Could you check a few things on this drawing? It's one solid part, dimensions in mm from its lowest x, y, z. A direction names the side the tool comes from. Give positions to 0.01 mm unless a question says otherwise; leave off trailing zeros. Order: outer loops, then holes, each group sorted by start corner. A loop starts at its lowest first (then second) coordinate and runs counter-clockwise, first axis right, second up. Notation, with made-up numbers: M 74,-28.75 L 116,-28.75 A24 cw 116,7.25 Z; hole C 4,12 d9. An arc over 180 degrees is marked long. Return JSON: item names as keys, results as strings. Group by question number.
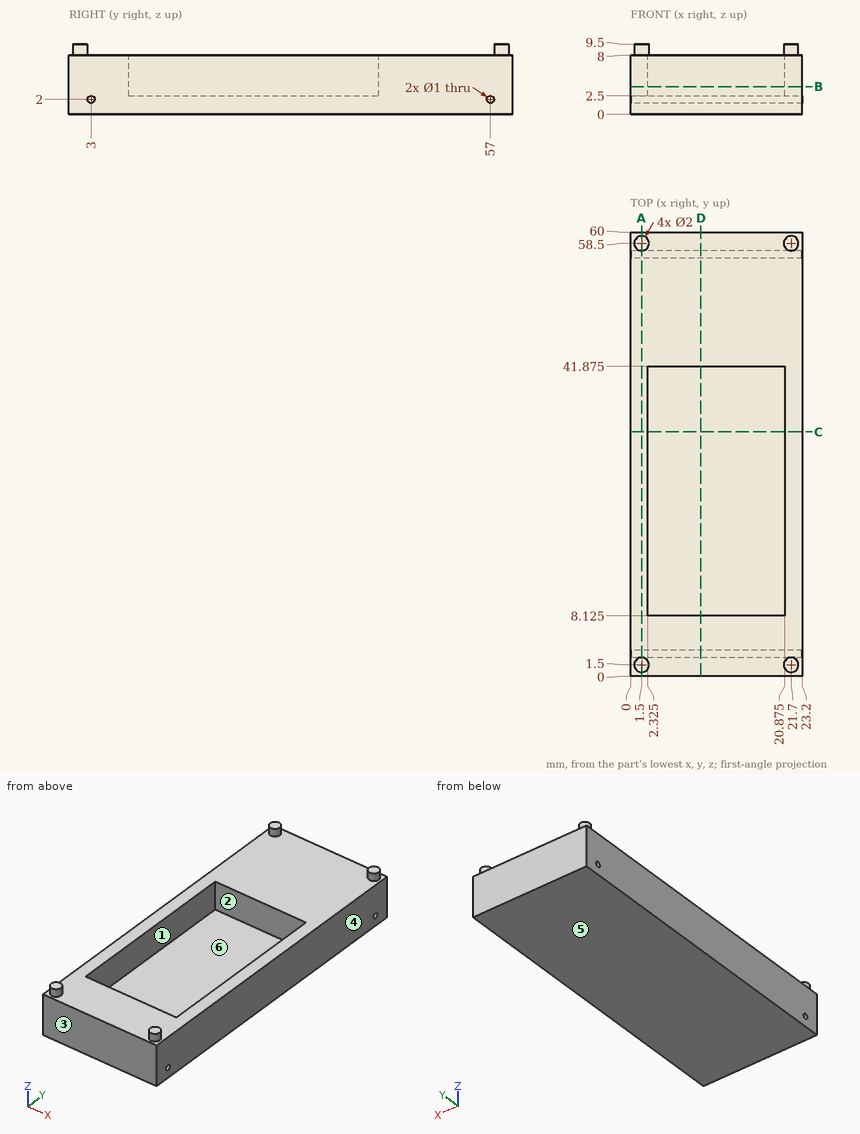
1. For pin 1 (4 mm diameter, centred on x = 16.5, y = 12.5, fed in from +Z), with a flat end and sliding along its axis, tell me the tip position at first contact or that it passes through.
2. I need wall thicknesses on L1, parallel to Y at x = 14.5, z = 2; L2, parallel to X at y = 18.5, z = 6 (3 decimals); L3, parallel to Y at x = 17.25, z = 7.5 (3 decimals). Which ranges of each line are inside material? Lowest first, please. Write a range as from..to.
3. If we mould it in two halves opening along Y, with no side actions, what happens to the marked faces 1, 2, 3 and 4? For each: pulls with the +Y half, pulls with the -Y half, needs draft (parallel to the pull), parting line crosses it, or undercut.
4. Imagine slicing it at B-B, the plane z = 3.75. Please give me the cut outline in (x, y) (3 decimals).
5. Imagine slicing it at A-A, the plane x = 1.5. Please give me the cut outline in (y, z).
6. Imagine slicing it at D-D, the plane x = 9.5. Please give me the cut outline in (y, z) (3 decimals).
7. Which directions (+Z, -Z, +X, -X, +Y, -Y) give clear straight access to the entire face, cutting with the end or side of a thin tool? Please do the marked faces 5 and 6.
8. Imagine slicing it at C-C, the plane y = 33. Please give me the cut outline in (x, z) (3 decimals), plus the area to 3 significant figures.
Values:
{
 "1": {"pin 1": "stops at z = 2.5"},
 "2": {"L1": "y = 0..2.5, 3.5..56.5, 57.5..60", "L2": "x = 0..2.325, 20.875..23.2", "L3": "y = 0..8.125, 41.875..60"},
 "3": {"face 1": "undercut", "face 2": "undercut", "face 3": "pulls with the -Y half", "face 4": "needs draft"},
 "4": {"outline": "M 0,0 L 23.2,0 L 23.2,60 L 0,60 Z; hole M 2.325,8.125 L 20.875,8.125 L 20.875,41.875 L 2.325,41.875 Z"},
 "5": {"outline": "M 0,0 L 60,0 L 60,8 L 59.5,8 L 59.5,9.5 L 57.5,9.5 L 57.5,8 L 2.5,8 L 2.5,9.5 L 0.5,9.5 L 0.5,8 L 0,8 Z; hole C 3,2 d1; hole C 57,2 d1"},
 "6": {"outline": "M 0,0 L 60,0 L 60,8 L 41.875,8 L 41.875,2.5 L 8.125,2.5 L 8.125,8 L 0,8 Z; hole C 3,2 d1; hole C 57,2 d1"},
 "7": {"face 5": "-Z, +X, -X, +Y, -Y", "face 6": "+Z"},
 "8": {"outline": "M 0,0 L 23.2,0 L 23.2,8 L 20.875,8 L 20.875,2.5 L 2.325,2.5 L 2.325,8 L 0,8 Z", "area": "83.6 mm²"}
}
